```python
from build123d import *

# Parameters (mm, degrees)
SKETCH_1_W                       = 195
SKETCH_1_H                       = 130
SM_BASE_FLANGE_1_DEPTH           = 3
SM_EDGE_FLANGE_1_STRIP_W         = 13.4732
SM_EDGE_FLANGE_1_STRIP_H         = 3
SM_EDGE_FLANGE_1_STRIP_CUT_DEPTH = 195
SM_EDGE_FLANGE_1_DEPTH           = 195
SM_EDGE_FLANGE_2_STRIP_W         = 13.4732
SM_EDGE_FLANGE_2_STRIP_H         = 3
SM_EDGE_FLANGE_2_STRIP_CUT_DEPTH = 195
SM_EDGE_FLANGE_2_DEPTH           = 195
SKETCH_12_R                      = 2
CUT_EXTRUDE_1_DEPTH              = 10
SKETCH_13_R                      = 2
CUT_EXTRUDE_2_DEPTH              = 10
CUT_EXTRUDE_3_REACH              = 119.899
SKETCH_14_R                      = 7.5


# Sheet-metal steps are written as plain solids
with BuildPart() as part:
    # Sketch 1 → 基体-法兰1 (new body)
    with BuildSketch(Plane(origin=(0, 0, 0), x_dir=(1, 0, 0), z_dir=(0, 1, 0))):
        Rectangle(SKETCH_1_W, SKETCH_1_H)
    extrude(amount=-SM_BASE_FLANGE_1_DEPTH)

    # 边线-法兰1 strip (across the edge) → 边线-法兰1 strip cut (cut)
    with BuildSketch(Plane(origin=(-97.5, 0, 65), x_dir=(0, 0, -1), z_dir=(1, 0, 0))):
        with Locations((-3, -1.5)):
            Rectangle(SM_EDGE_FLANGE_1_STRIP_W, SM_EDGE_FLANGE_1_STRIP_H)
    extrude(amount=SM_EDGE_FLANGE_1_STRIP_CUT_DEPTH, mode=Mode.SUBTRACT)

    # 边线-法兰1 section (across the edge) → 边线-法兰1 (add)
    with BuildSketch(Plane(origin=(-97.5, 0, 65), x_dir=(0, 0, -1), z_dir=(1, 0, 0))):
        with BuildLine():
            Line((0, 0.7366), (0, 10))
            Line((0, 10), (3, 10))
            Line((3, 10), (3, 0.7366))
            ThreePointArc((3, 0.7366), (3.215745145, 0.215745145), (3.7366, 0))
            Line((3.7366, 0), (3.7366, -3))
            ThreePointArc((3.7366, -3), (1.094424801, -1.905575199), (0, 0.7366))
        make_face()
    extrude(amount=SM_EDGE_FLANGE_1_DEPTH)

    # 边线-法兰2 strip (across the edge) → 边线-法兰2 strip cut (cut)
    with BuildSketch(Plane(origin=(-97.5, -3, -65), x_dir=(0, 0, 1), z_dir=(1, 0, 0))):
        with Locations((-3, -1.5)):
            Rectangle(SM_EDGE_FLANGE_2_STRIP_W, SM_EDGE_FLANGE_2_STRIP_H)
    extrude(amount=SM_EDGE_FLANGE_2_STRIP_CUT_DEPTH, mode=Mode.SUBTRACT)

    # 边线-法兰2 section (across the edge) → 边线-法兰2 (add)
    with BuildSketch(Plane(origin=(-97.5, -3, -65), x_dir=(0, 0, 1), z_dir=(1, 0, 0))):
        with BuildLine():
            Line((0, 0.7366), (0, 10))
            Line((0, 10), (3, 10))
            Line((3, 10), (3, 0.7366))
            ThreePointArc((3, 0.7366), (3.215745145, 0.215745145), (3.7366, 0))
            Line((3.7366, 0), (3.7366, -3))
            ThreePointArc((3.7366, -3), (1.094424801, -1.905575199), (0, 0.7366))
        make_face()
    extrude(amount=SM_EDGE_FLANGE_2_DEPTH)

    # 草图12 → 切除-拉伸1 (cut)
    with BuildSketch(Plane.XY.offset(65)):
        with Locations((-55, 5)):
            Circle(SKETCH_12_R)
        with Locations(Location((55, 5, 0), (0, 0, 180))):
            Circle(SKETCH_12_R)
    extrude(amount=-CUT_EXTRUDE_1_DEPTH, mode=Mode.SUBTRACT)

    # 草图13 → 切除-拉伸2 (cut)
    with BuildSketch(Plane(origin=(0, 0, -65), x_dir=(-1, 0, 0), z_dir=(0, 0, -1))):
        with Locations(Location((-55, -8, 0), (0, 0, 90))):
            Circle(SKETCH_13_R)
        with Locations(Location((55, -8, 0), (0, 0, 270))):
            Circle(SKETCH_13_R)
    extrude(amount=-CUT_EXTRUDE_2_DEPTH, mode=Mode.SUBTRACT)

    # 草图14 → 切除-拉伸3 (cut, up to next)
    with BuildSketch(Plane.XZ.offset(3), mode=Mode.PRIVATE) as cut_extrude_3_sk1:
        with Locations(Location((65, -32, 0), (0, 0, 270))):
            Circle(SKETCH_14_R)
    cut_extrude_3_tool1 = extrude(cut_extrude_3_sk1.sketch, amount=-CUT_EXTRUDE_3_REACH, mode=Mode.PRIVATE) & part.part
    add(cut_extrude_3_tool1.solids().sort_by_distance((65, -3, -32))[0], mode=Mode.SUBTRACT)


solid = part.part
```
Work out the finished part from the listing and answer in its coordinate system (mm). A direction names the side the tool comes from. Give positions to 0.01 mm unless a question says otherwise; leave off trailing zeros. Order: outer loops, then holes, each group sorted by start corner. A loop starts at its lowest first (then second) coordinate and runs counter-clockwise, first axis right, second up.
1. Each of these flat-tipped pins is pushed along its axis until it touches: P1, Ø2, axis at x = 45.5, z = -29.5, coming from the -Y side; P2, Ø5, axis at x = -55, y = -8, coming from the +Z side; P3, Ø2, axis at x = -59.5, y = 0, coming from the -Z side. Where does it stop, or does it pass through?
Result sheet:
P1: stops at y = -3
P2: stops at z = -62
P3: stops at z = -63.81
2. For faces 5 (the flat face through (-1, 5, 62)), 6 (the flat face through (-1, -3, -1)), 7 (the cylindrical face through (70.1, -1.5, -26.5)), determine the directions among +Z, -Z, +X, -X, +Y, -Y from which every point of the face is accessible in a straight line to the end or side of a thin tool.
Result sheet:
face 5: -Z, +X, -X, +Y
face 6: +Z, +X, -X, -Y
face 7: +Y, -Y
3. Section B-B, the plane y = -8 is taken. Determine the outline of the cut face in (x, z).
Result sheet:
outline: (-97.5, -65) - (-57, -65) - (-57, -62) - (-97.5, -62) - close; (-53, -65) - (53, -65) - (53, -62) - (-53, -62) - close; (57, -65) - (97.5, -65) - (97.5, -62) - (57, -62) - close
4. Section A-A, the plane x = -55 is taken. Determine the outline of the cut face in (y, z), and give its area (3 significant figures).
Result sheet:
outline: (-13, -65) - (-10, -65) - (-10, -62) - (-13, -62) - close; (-6, -65) - (-3.74, -65) arc R3.74 ccw to (0, -61.26) - (0, 61.26) arc R0.74 cw to (0.74, 62) - (3, 62) - (3, 65) - (0.74, 65) arc R3.74 ccw to (-3, 61.26) - (-3, -61.26) arc R0.74 cw to (-3.74, -62) - (-6, -62) - close; (7, 62) - (10, 62) - (10, 65) - (7, 65) - close
area: 420 mm2
5. Straight lines are drawn through the part: L1, parallel to X at y = -8, z = -62.6; L2, parallel to Y at x = 28.5, z = -16; L3, parallel to Z at x = 10, y = 6. For each, find the intervals that lie inside material, in ascending order.
Result sheet:
L1: x = -97.5 to -57, -53 to 53, 57 to 97.5
L2: y = -3 to 0
L3: z = 62 to 65
6. The mould has two halves that part along X. Classify faces 1 (the flat face through (-97.5, -2, 0)), 2 (the flat face through (-1, 0, -1)), 3 (the flat face through (97.5, -2, 0)), 4 (the cylindrical face through (-57, 5, 64)): released by +X, released by -X, zero draft, split by the parting line, or undercut.
Result sheet:
face 1: released by -X
face 2: zero draft
face 3: released by +X
face 4: undercut
7. Section C-C, the plane x = 65 is taken. Determine the outline of the cut face in (y, z).
Result sheet:
outline: (-13, -65) - (-3.74, -65) arc R3.74 ccw to (0, -61.26) - (0, -39.5) - (-3, -39.5) - (-3, -61.26) arc R0.74 cw to (-3.74, -62) - (-13, -62) - close; (-3, -24.5) - (0, -24.5) - (0, 61.26) arc R0.74 cw to (0.74, 62) - (10, 62) - (10, 65) - (0.74, 65) arc R3.74 ccw to (-3, 61.26) - close
8. Section D-D, the plane z = -32 is taken. Determine the outline of the cut face in (x, y).
Result sheet:
outline: (-97.5, -3) - (57.5, -3) - (57.5, 0) - (-97.5, 0) - close; (72.5, -3) - (97.5, -3) - (97.5, 0) - (72.5, 0) - close
